The model under review builds one solid part; all positions refer to its coordinate system, in mm. Give positions to 0.01 mm unless a question says otherwise; leave off trailing zeros. Order: outer loops, then holes, each group sorted by start corner. A loop starts at its lowest first (then second) coordinate and runs counter-clockwise, first axis right, second up. Notation, with made-up numbers: (-29, 83) - (-25, 83) arc R28 cw to (-25, 101) - close; hole circle Ø10 at (-39.5, 20.5). An arc over 180 degrees is marked (long way). Put each result on its own line as item: value.
```python
from build123d import *

# Parameters (mm, degrees)
BOSS_EXTRUDE1_DEPTH  = 5.6388
SKETCH2_W            = 76.2
SKETCH2_H            = 6.35
CUT_EXTRUDE1_DEPTH   = 6.6388
LPATTERN1_COUNT      = 5
LPATTERN1_PITCH      = 12.7
LPATTERN1_COUNT_DIR2 = 3
LPATTERN1_PITCH_DIR2 = 100
SKETCH3_W            = 120.65
SKETCH3_H            = 41.75
CUT_EXTRUDE2_DEPTH   = 6.6388


with BuildPart() as part:
    # Sketch1 → Boss-Extrude1 (new body)
    with BuildSketch(Plane(origin=(0, 0, 0), x_dir=(1, 0, 0), z_dir=(0, 1, 0))):
        Polygon((-185, -73.025), (185, -73.025), (185, -6.825), (185, 3.175), (175, 3.175), (-175, 3.175), (-185, 3.175), (-185, -6.825), align=None)
    extrude(amount=BOSS_EXTRUDE1_DEPTH)

    # Sketch2 → Cut-Extrude1 (cut, through all)
    with BuildSketch(Plane(origin=(0, 5.6388, 0), x_dir=(1, 0, 0), z_dir=(0, 1, 0))):
        with Locations((-96.1, -59.85)):
            Rectangle(SKETCH2_W, SKETCH2_H)
    cut_extrude1 = extrude(amount=-CUT_EXTRUDE1_DEPTH, mode=Mode.SUBTRACT)

    # LPattern1: Cut-Extrude1 5 × 3
    with Locations(*[(j * LPATTERN1_PITCH_DIR2, 0, -i * LPATTERN1_PITCH) for i in range(LPATTERN1_COUNT) for j in range(LPATTERN1_COUNT_DIR2) if (i, j) != (0, 0)]):
        add(cut_extrude1, mode=Mode.SUBTRACT)

    # Sketch3 → Cut-Extrude2 (cut, through all)
    with BuildSketch(Plane(origin=(0, 5.6388, 0), x_dir=(1, 0, 0), z_dir=(0, 1, 0))):
        with Locations((-118.325, -52.15)):
            Rectangle(SKETCH3_W, SKETCH3_H)
    extrude(amount=-CUT_EXTRUDE2_DEPTH, mode=Mode.SUBTRACT)


solid = part.part
```
(1) Take a section at B-B, the plane x = 121.5. Write out the cut boundary in (y, z) (3 decimals), then the cut area to 3 significant figures.
The answers:
outline: (0, -3.175) - (5.639, -3.175) - (5.639, 5.875) - (0, 5.875) - close; (0, 12.225) - (5.639, 12.225) - (5.639, 18.575) - (0, 18.575) - close; (0, 24.925) - (5.639, 24.925) - (5.639, 31.275) - (0, 31.275) - close; (0, 37.625) - (5.639, 37.625) - (5.639, 43.975) - (0, 43.975) - close; (0, 50.325) - (5.639, 50.325) - (5.639, 56.675) - (0, 56.675) - close; (0, 63.025) - (5.639, 63.025) - (5.639, 73.025) - (0, 73.025) - close
area: 251 mm^2
(2) Take a section at A-A, the plane x = -106. Write out the cut boundary in (y, z) (3 decimals), then the cut area to 3 significant figures.
The answers:
outline: (0, -3.175) - (5.639, -3.175) - (5.639, 5.875) - (0, 5.875) - close; (0, 12.225) - (5.639, 12.225) - (5.639, 18.575) - (0, 18.575) - close; (0, 24.925) - (5.639, 24.925) - (5.639, 31.275) - (0, 31.275) - close
area: 123 mm^2
(3) Clearance check with a flat-ended pin moving along its axis: pin 1 Ø12 at (x, z) = (-67.5, 50) entering from -Y. State where the tip first meets the part, or that it passes through.
The answers:
pin 1: through
(4) Wall thickness on L1, parallel to Z at x = -124.5, y = 1.7 (3 decimals); L2, parallel to X at y = 1, z = 12; L3, parallel to Z at x = -22.5, y = 1.65 (3 decimals): over which ranges is each line inside the solid? List them lowest first.
The answers:
L1: -3.175 to 5.875, 12.225 to 18.575, 24.925 to 31.275
L2: -185 to -134.2, -58 to -34.2, 42 to 65.8, 142 to 185
L3: -3.175 to 5.875, 12.225 to 18.575, 24.925 to 31.275, 37.625 to 43.975, 50.325 to 56.675, 63.025 to 73.025
(5) Take a section at C-C, the plane z = 68.5. Write out the cut boundary in (x, y), then the cut area to 3 significant figures.
The answers:
outline: (-185, 0) - (-178.65, 0) - (-178.65, 5.64) - (-185, 5.64) - close; (-58, 0) - (185, 0) - (185, 5.64) - (-58, 5.64) - close
area: 1,410 mm^2
(6) Take a section at D-D, the plane y = 1.8. Count the separate pieces of the cut face and the enclosed holes in it, then the cut area to 3 significant figures.
The answers:
separate pieces: 1
enclosed holes: 12
area: 17,400 mm^2
